from build123d import *

# Parameters (mm, degrees)
F1_DEPTH = 25.4
F2_W     = 50.8
F2_H     = 50.8
F3_DEPTH = 127


# Not quite as in the source:
# - a feature of the source that left no trace in its solid (it failed there, or was rolled back) is left out
# - the program builds the solid bodies; features that only make, move or delete a surface that nothing else refers to are left out


with BuildPart() as f1:
    # F0 (on Front) → F1 (new body, symmetric)
    with BuildSketch(Plane.XZ):
        Polygon((0, -50.8), (0, 0), (-203.2, 0), (-203.2, 965.2), (-254, 965.2), (-254, -50.8), align=None)
    extrude(amount=F1_DEPTH, both=True)

    # F2 (on face) → F3 (join)
    with BuildSketch(Plane.XZ.offset(25.4)):
        with Locations((-228.6, 939.8)):
            Rectangle(F2_W, F2_H)
    extrude(amount=F3_DEPTH)

    # F4: F1 across plane


with BuildPart() as f1_1:
    add(f1.part)
    add(f1.part.mirror(Plane.XZ))


solid = f1_1.part
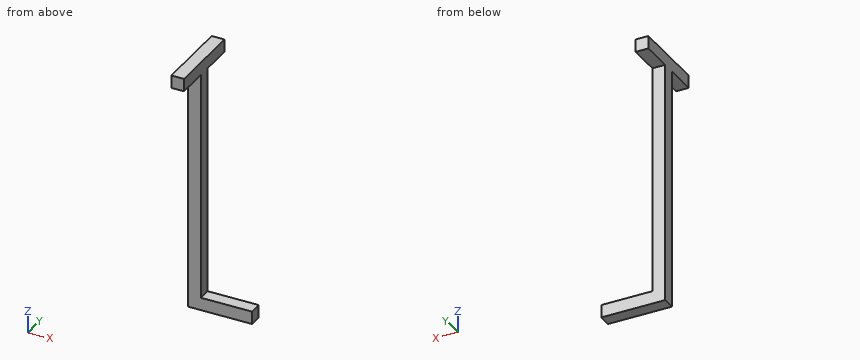
Could you check a few things on this model? Use its own coordinates, in mm. Give positions to 0.01 mm unless a question says otherwise; leave off trailing zeros. Order: outer loops, then holes, each group sorted by start corner. A loop starts at its lowest first (then second) coordinate and runs counter-clockwise, first axis right, second up. Notation, with made-up numbers: (74.25, -10.75) - (113.25, -10.75) arc R13 cw to (113.25, -0.75) - close; hole circle Ø2 at (-14.5, 80). An arc over 180 degrees is marked (long way). One line per item, written item: value. Start each with the question number.
1. If I drill on probe 1 along Y at (x, z) = (-214.5, 117.5); probe 2 along Z at (x, y) = (-223, 128); probe 3 along Z at (x, y) = (-59.5, 0), over which ranges is the centre line in solid material (lowest first)?
2. Imagine slicing it at D-D on x = -37. List the corners of the cut face in (y, z) for me, plus the area to 3 significant figures.
3. Imagine slicing it at C-C on z = 97.5. List the corners of the cut face in (x, y) for me.
4. Imagine slicing it at A-A on x = -213.5. List the corners of the cut face in (y, z) for me, plus the area to 3 significant figures.
5. Imagine slicing it at B-B on y = 6. List the corners of the cut face in (x, z) for me, plus the area to 3 significant figures.
6. For P1, Ø10, axis at x = -199, y = 81, coming from the -Z side; P2, Ø2, axis at x = -216.5, z = 560, coming from the +Y side, each with a flat end and sliding along its axis, tell me the tip position at first contact or that it passes through.
Values:
1. probe 1: -25.4 to 25.4
1. probe 2: 914.4 to 965.2
1. probe 3: -50.8 to 0
2. outline: (-25.4, -50.8) - (25.4, -50.8) - (25.4, 0) - (-25.4, 0) - close
2. area: 2,580 mm²
3. outline: (-254, -25.4) - (-203.2, -25.4) - (-203.2, 25.4) - (-254, 25.4) - close
4. outline: (-152.4, 914.4) - (-25.4, 914.4) - (-25.4, -50.8) - (25.4, -50.8) - (25.4, 914.4) - (152.4, 914.4) - (152.4, 965.2) - (-152.4, 965.2) - close
4. area: 64,500 mm²
5. outline: (-254, -50.8) - (0, -50.8) - (0, 0) - (-203.2, 0) - (-203.2, 965.2) - (-254, 965.2) - close
5. area: 61,900 mm²
6. P1: z = 914.4
6. P2: y = 25.4
